Autodesk Inventor part; units mm, degrees
ref_plane "YZ Plane" through (0, 0, 0) normal (1, 0, 0) x (0, 1, 0)
ref_plane "XZ Plane" through (0, 0, 0) normal (0, 1, 0) x (-1, 0, 0)
ref_plane "XY Plane" through (0, 0, 0) normal (0, 0, 1) x (1, 0, 0)
sketch "スケッチ1" plane through (0, 0, 0) normal (0, 0, 1) x (1, 0, 0)
  circle A0 centre (-165.8946, -3.3102) radius 1.5
  circle A1 centre (-136.5368, 15.7454) radius 1.5
  circle A2 centre (-82.4879, 34.801) radius 1.5
  circle A3 centre (-77.8211, 53.8566) radius 1.5
  circle A4 centre (-107.1789, 34.801) radius 1.5
  circle A5 centre (-110.4783, 13.7882) radius 1.5
  circle A6 centre (-138.4687, -7.2246) radius 1.5
  circle A7 centre (-184.7359, -19.7422) radius 1.5
  circle A8 centre (-173.2477, -31.458) radius 1.5
  circle A9 centre (-44.4492, 64.0137) radius 1.5
  circle A10 centre (-64.4423, 49.0046) radius 1.5
  circle A11 centre (-60.4494, 64.5064) radius 1.5
  line L0 (-64.2741, 70.3989) -> (-190.1939, -11.3332)
  arc A12 (-190.1939, -11.3332) -> (-190.9729, -27.5907) centre (-184.7359, -19.7422) ccw
  line L1 (-190.9729, -27.5907) -> (-178.2249, -37.7212)
  arc A13 (-178.2249, -37.7212) -> (-168.4448, -37.8558) centre (-173.2477, -31.458) ccw
  line L2 (-168.4448, -37.8558) -> (-40.2316, 58.3956)
  arc A14 (-40.2316, 58.3956) -> (-44.233, 71.0354) centre (-44.4492, 64.0137) ccw
  line L3 (-44.233, 71.0354) -> (-60.2332, 71.5281)
  arc A15 (-60.2332, 71.5281) -> (-64.2741, 70.3989) centre (-60.4494, 64.5064) ccw
  arc A16 (-161.5407, -4.4476) -> (-168.8524, 0.0812) centre (-165.8946, -3.3102) ccw
  arc A17 (-187.6936, -16.3507) -> (-187.9489, -22.8928) centre (-184.7359, -19.7422) ccw
  arc A18 (-176.4608, -34.6086) -> (-168.8938, -32.5954) centre (-173.2477, -31.458) ccw
  line L4 (-187.6936, -16.3507) -> (-168.8524, 0.0812)
  line L5 (-161.5407, -4.4476) -> (-168.8938, -32.5954)
  line L6 (-187.9489, -22.8928) -> (-176.4608, -34.6086)
  point P0 (0, 0)
  point P1 (0, 0)
  dimension "d0" = 3
  dimension "d1" = 3
  dimension "d2" = 3
extrude "押し出し1" add sketch "スケッチ1" along normal blind 3 contours L5 A18 L6 A17 L4 A16
properties part number "アーム抑えツイン1" material "ポリカーボネート、クリア"
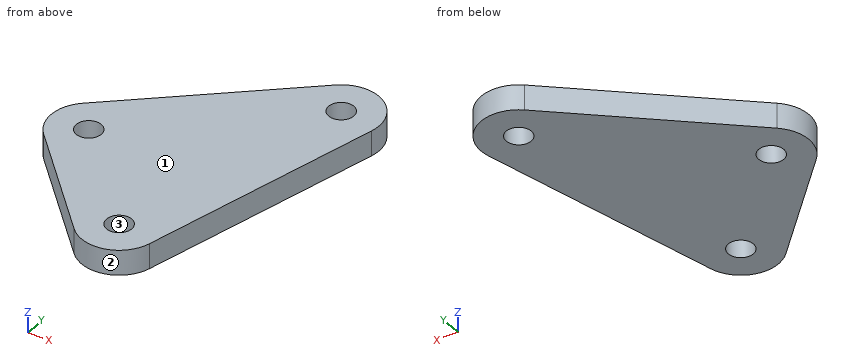
CAD build for the part. Positions are in the model's coordinates, mm. Face numbers are marked on the shaded views. Round coordinates to 2 decimals unless told otherwise and drop trailing zeros. Order: outer loops, then holes, each group sorted by start corner. A loop starts at its lowest first (then second) coordinate and runs counter-clockwise, first axis right, second up. Notation, with made-up numbers: (54.25, -4) -> (82.25, -4) arc R7 cw to (82.25, 4) -> close; hole circle Ø8 at (-2.75, -4.5). An arc over 180 degrees is marked (long way). Write each question's results on one line, items separated by ' | '.
1. Pull direction X, two halves, no side cores. Call the marked faces 1, 2 and 3: pulls with the +X half, pulls with the -X half, needs draft (parallel to the pull), parting line crosses it, or undercut.
Findings below:
face 1: needs draft | face 2: parting line crosses it | face 3: undercut
2. Wall check: line 1 along X through (y, z) = (-19, 0.4); line 2 along X through (y, z) = (-2.5, 2.25); line 3 along Y through (x, z) = (-184.5, 1.15). Give the ranges that are in metal, low to high. Write a range as [from, to].
Findings below:
line 1: x = [-189.17, -186.04], [-183.43, -165.34] | line 2: x = [-171.81, -167.16], [-164.63, -161.47] | line 3: y = [-26.41, -21.22], [-18.26, -13.57]
3. Cut at D-D (x = -173.75). Give the cut face in (y, z).
Findings below:
outline: (-35.93, 0) -> (-32.87, 0) -> (-32.87, 3) -> (-35.93, 3) -> close; (-30.04, 0) -> (-4.19, 0) -> (-4.19, 3) -> (-30.04, 3) -> close
4. Cut at C-C (y = -7). Give the cut face in (x, z), plus the area to 3 significant figures.
Findings below:
outline: (-176.97, 0) -> (-162.21, 0) -> (-162.21, 3) -> (-176.97, 3) -> close | area: 44.3 mm²
5. Cut at B-B (x = -165). Give the cut face in (y, z), plus the area to 3 significant figures.
Findings below:
outline: (-17.69, 0) -> (-4.51, 0) -> (-4.51, 3) -> (-17.69, 3) -> close; (-2.11, 0) -> (1.1, 0) -> (1.1, 3) -> (-2.11, 3) -> close | area: 49.1 mm²
6. Cut at A-A (z = 1.75). Give the cut face in (x, y).
Findings below:
outline: (-187.95, -22.89) -> (-176.46, -34.61) arc R4.5 ccw to (-168.89, -32.6) -> (-161.54, -4.45) arc R4.5 ccw to (-168.85, 0.08) -> (-187.69, -16.35) arc R4.5 ccw to start; hole circle Ø3 at (-184.74, -19.74); hole circle Ø3 at (-173.25, -31.46); hole circle Ø3 at (-165.89, -3.31)
7. Flat gauge pins, fed straight in: P1, Ø1.5, axis at x = -167, z = 2.5, coming from the +Y side; P2, Ø1.5, axis at x = -176, z = 2.5, coming from the -Y side. Where does each tip first touch, or does it go through?
Findings below:
P1: stops at y = 1.18 | P2: stops at y = -35.49
